from build123d import *

# Parameters (mm, degrees)
SKETCH1_W           = 100
SKETCH1_H           = 8
BOSS_EXTRUDE1_DEPTH = 7
SKETCH3_W           = 100
SKETCH3_H           = 20
BOSS_EXTRUDE2_DEPTH = 2
SKETCH2_W           = 100
SKETCH2_H           = 3.1
CUT_EXTRUDE1_DEPTH  = 5.7
FILLET1_R           = 1
SKETCH4_R           = 2.1
CUT_EXTRUDE2_DEPTH  = 2
FILLET2_R           = 0.75
CHAMFER1_SIZE       = 0.75


with BuildPart() as part:
    # Sketch1 → Boss-Extrude1 (new body)
    with BuildSketch(Plane(origin=(0, 0, 0), x_dir=(1, 0, 0), z_dir=(0, 1, 0))):
        Rectangle(SKETCH1_W, SKETCH1_H)
    extrude(amount=BOSS_EXTRUDE1_DEPTH)

    # Sketch3 → Boss-Extrude2 (add)
    with BuildSketch(Plane(origin=(0, 0, 0), x_dir=(1, 0, 0), z_dir=(0, 1, 0))):
        Rectangle(SKETCH3_W, SKETCH3_H)
    extrude(amount=BOSS_EXTRUDE2_DEPTH)

    # Sketch2 → Cut-Extrude1 (cut)
    with BuildSketch(Plane(origin=(0, 7, 0), x_dir=(1, 0, 0), z_dir=(0, 1, 0))):
        Rectangle(SKETCH2_W, SKETCH2_H)
    extrude(amount=-CUT_EXTRUDE1_DEPTH, mode=Mode.SUBTRACT)

    # Fillet1
    fillet1_edges = [part.edges().sort_by_distance(p)[0] for p in [
        (-50, 7, -2.775),
        (0, 7, 4),
        (50, 7, -2.775),
        (-50, 7, 2.775),
        (0, 7, -1.55),
        (0, 7, 1.55),
        (50, 7, 2.775),
        (0, 7, -4),
    ]]
    fillet(fillet1_edges, radius=FILLET1_R)

    # Sketch4 → Cut-Extrude2 (cut)
    with BuildSketch(Plane(origin=(0, 2, 0), x_dir=(1, 0, 0), z_dir=(0, 1, 0))):
        with Locations(Location((-45.9, 7, 0), (0, 0, 270))):
            Circle(SKETCH4_R)
        with Locations(Location((-45.9, -7, 0), (0, 0, 270))):
            Circle(SKETCH4_R)
        with Locations(Location((45.9, 7, 0), (0, 0, 270))):
            Circle(SKETCH4_R)
        with Locations(Location((45.9, -7, 0), (0, 0, 270))):
            Circle(SKETCH4_R)
    extrude(amount=-CUT_EXTRUDE2_DEPTH, mode=Mode.SUBTRACT)

    # Fillet2
    fillet2_edges = [part.edges().sort_by_distance(p)[0] for p in [
        (-50, 2, -7),
        (50, 2, -7),
        (0, 2, -10),
        (50, 2, 7),
        (-50, 2, 7),
        (0, 2, 10),
    ]]
    fillet(fillet2_edges, radius=FILLET2_R)

    # Chamfer1
    # the kernel refuses this chamfer: 0.75 mm, written as the material it adds along each edge
    with BuildSketch(Plane(origin=(49.25, 2, -4), x_dir=(0, -0.02749587661058648, -0.9996219169112968), z_dir=(-1, 0, 0)), Plane(origin=(-49.25, 2, 4), x_dir=(0, -0.02749587661058648, 0.9996219169112968), z_dir=(1, 0, 0))) as chamfer1_piece_1:
        Polygon((CHAMFER1_SIZE * 0.999621916911, -CHAMFER1_SIZE * 0.0274958766106), (-CHAMFER1_SIZE * 0.0274958766106, -CHAMFER1_SIZE * 0.999621916911), (0, 0), align=None)
    extrude(amount=98.5)
    with BuildSketch(Plane(origin=(49.25, 1.25, -4), x_dir=(-0.8425066666450713, -0.5386859165215022, 0), z_dir=(-0.5386859165215022, 0.8425066666450713, 0))) as chamfer1_piece_2_section:
        Polygon((0.75, -CHAMFER1_SIZE), (0.75 + CHAMFER1_SIZE, 0), (0.75, 0), align=None)
    chamfer1_piece_2 = revolve(axis=Axis((49.25, 1.25, -4), (0, 0, 1)), revolution_arc=237.405771779, mode=Mode.PRIVATE)
    chamfer1_piece_2 = split(chamfer1_piece_2, bisect_by=Plane(origin=(50, 1.825736319, -4.33178547), z_dir=(-1, 0, 0)), keep=Keep.TOP, mode=Mode.PRIVATE)
    chamfer1_piece_2 = split(chamfer1_piece_2, bisect_by=Plane(origin=(49.825736319, 0, -4.33178547), z_dir=(0, 1, 0)), keep=Keep.TOP, mode=Mode.PRIVATE)
    add(chamfer1_piece_2)
    with BuildSketch(Plane(origin=(49.25, 1.25, 4), x_dir=(-0.8425066666450713, -0.5386859165215022, 0), z_dir=(-0.5386859165215022, 0.8425066666450713, 0))) as chamfer1_piece_3_section:
        Polygon((0.75 + CHAMFER1_SIZE, 0), (0.75, CHAMFER1_SIZE), (0.75, 0), align=None)
    chamfer1_piece_3 = revolve(axis=Axis((49.25, 1.25, 4), (0, 0, 1)), revolution_arc=237.405771779, mode=Mode.PRIVATE)
    chamfer1_piece_3 = split(chamfer1_piece_3, bisect_by=Plane(origin=(50, 1.825736319, 4.33178547), z_dir=(-1, 0, 0)), keep=Keep.TOP, mode=Mode.PRIVATE)
    chamfer1_piece_3 = split(chamfer1_piece_3, bisect_by=Plane(origin=(49.825736319, 0, 4.33178547), z_dir=(0, 1, 0)), keep=Keep.TOP, mode=Mode.PRIVATE)
    add(chamfer1_piece_3)
    with BuildSketch(Plane(origin=(-49.25, 1.25, 4), x_dir=(0, 1, 0), z_dir=(1, 0, 0))) as chamfer1_piece_4_section:
        Polygon((0.75, CHAMFER1_SIZE), (0.75 + CHAMFER1_SIZE, 0), (0.75, 0), align=None)
    chamfer1_piece_4 = revolve(axis=Axis((-49.25, 1.25, 4), (0, 0, 1)), revolution_arc=237.405771779, mode=Mode.PRIVATE)
    chamfer1_piece_4 = split(chamfer1_piece_4, bisect_by=Plane(origin=(-50, 1.825736319, 4.33178547), z_dir=(1, 0, 0)), keep=Keep.TOP, mode=Mode.PRIVATE)
    chamfer1_piece_4 = split(chamfer1_piece_4, bisect_by=Plane(origin=(-49.825736319, 0, 4.33178547), z_dir=(0, 1, 0)), keep=Keep.TOP, mode=Mode.PRIVATE)
    add(chamfer1_piece_4)
    with BuildSketch(Plane(origin=(-49.25, 1.25, -4), x_dir=(0, 1, 0), z_dir=(1, 0, 0))) as chamfer1_piece_5_section:
        Polygon((0.75, -CHAMFER1_SIZE), (0.75 + CHAMFER1_SIZE, 0), (0.75, 0), align=None)
    chamfer1_piece_5 = revolve(axis=Axis((-49.25, 1.25, -4), (0, 0, 1)), revolution_arc=237.405771779, mode=Mode.PRIVATE)
    chamfer1_piece_5 = split(chamfer1_piece_5, bisect_by=Plane(origin=(-50, 1.825736319, -4.33178547), z_dir=(1, 0, 0)), keep=Keep.TOP, mode=Mode.PRIVATE)
    chamfer1_piece_5 = split(chamfer1_piece_5, bisect_by=Plane(origin=(-49.825736319, 0, -4.33178547), z_dir=(0, 1, 0)), keep=Keep.TOP, mode=Mode.PRIVATE)
    add(chamfer1_piece_5)


solid = part.part
Source: CAD feature listing. Evaluate the final solid. Frame: model axes, mm. A direction names the side the tool comes from. Give positions to 0.01 mm unless a question says otherwise; leave off trailing zeros. Write each loop counter-clockwise with the first axis right and the second up, starting at its lowest first coordinate (ties: lowest second). Pieces come first, ordered by that corner, then holes. Notation, with made-up numbers: (25, 19) -> (75, 19) arc R31 ccw to (75, 54) -> close; hole circle Ø11 at (24, 51). An arc over 180 degrees is marked (long way). Return JSON: item names as keys, results as strings. Group by question number.
1. Mould query, pull axis X, two halves, no side actions, for faces 1 (the face through (48, 1, 7)), 2 (the face through (-1, 2, -7)), 3 (the face through (48, 1, -7)), 4 (the face through (50, 1, 0)). Classes: +X half, -X half, draft (parallel to the pull), parting line (faces both ways), or undercut.
2. Material intervals for line 1 (X direction, y = 1.05, z = -7); line 2 (Z direction, x = -10.5, y = 5); line 3 (Y direction, x = 6.5, z = 7.5), sorted ascending. Write a range as from..to.
3. Section C-C, the plane z = 7. Output: boundary loops of the cut face in (x, y), then the cut area to 3 significant figures.
4. Access query for faces 5 (the face through (-1, 4, 1.55)), 6 (the face through (-1, 2, 7)), 7 (the face through (1, 0, 0)). Directions: +Z, -Z, +X, -X, +Y, -Y. A direction counts if a zero-diameter tool reaches every point of the face in a straight line with its end or side. Return the directions, or none.
5. Section D-D, the plane x = 11.5. Output: boundary loops of the cut face in (y, z), then the cut area to 3 significant figures.
6. Section B-B, the plane y = 5. Output: boundary loops of the cut face in (x, z), then the cut area to 3 significant figures.
7. Pin query (flat end, axial travel): pin 1 Ø3.5 at (x, z) = (45.9, 7) entering from -Y; pin 2 Ø1.4 at (x, z) = (8, 7.5) entering from +Y; pin 3 Ø0.9 at (x, z) = (9, 0.5) entering from +Y; pin 4 Ø1.7 at (x, y) = (-22, 4.5) entering from +Z. Return the tip coordinate at first contact, or that it passes through.
8. Section A-A, the plane x = 45.9. Output: boundary loops of the cut face in (y, z), then the cut area to 3 significant figures.
Determined:
{
 "1": {"face 1": "undercut", "face 2": "draft", "face 3": "undercut", "face 4": "+X half"},
 "2": {"line 1": "x = -50..-48, -43.8..43.8, 48..50", "line 2": "z = -4..-1.55, 1.55..4", "line 3": "y = 0..2"},
 "3": {"outline": "(-50, 0) -> (-48, 0) -> (-48, 2) -> (-49.25, 2) arc R0.75 ccw to (-50, 1.25) -> close; (-43.8, 0) -> (43.8, 0) -> (43.8, 2) -> (-43.8, 2) -> close; (48, 0) -> (50, 0) -> (50, 1.25) arc R0.75 ccw to (49.25, 2) -> (48, 2) -> close", "area": "183 mm2"},
 "4": {"face 5": "+X, -X, +Y", "face 6": "+Z, +X, -X, +Y", "face 7": "+Z, -Z, +X, -X, -Y"},
 "5": {"outline": "(0, -10) -> (1.25, -10) arc R0.75 ccw to (2, -9.25) -> (2, -4.75) -> (2.75, -4) -> (6, -4) arc R1 ccw to (7, -3) -> (7, -2.55) arc R1 ccw to (6, -1.55) -> (1.3, -1.55) -> (1.3, 1.55) -> (6, 1.55) arc R1 ccw to (7, 2.55) -> (7, 3) arc R1 ccw to (6, 4) -> (2.75, 4) -> (2, 4.75) -> (2, 9.25) arc R0.75 ccw to (1.25, 10) -> (0, 10) -> close", "area": "61.8 mm2"},
 "6": {"outline": "(-50, -4) -> (50, -4) -> (50, -1.55) -> (-50, -1.55) -> close; (-50, 1.55) -> (50, 1.55) -> (50, 4) -> (-50, 4) -> close", "area": "490 mm2"},
 "7": {"pin 1": "passes through", "pin 2": "stops at y = 2", "pin 3": "stops at y = 1.3", "pin 4": "stops at z = 4"},
 "8": {"outline": "(0, -10) -> (1.25, -10) arc R0.75 ccw to (2, -9.25) -> (2, -9.1) -> (0, -9.1) -> close; (0, -4.9) -> (2, -4.9) -> (2, -4.75) -> (2.75, -4) -> (6, -4) arc R1 ccw to (7, -3) -> (7, -2.55) arc R1 ccw to (6, -1.55) -> (1.3, -1.55) -> (1.3, 1.55) -> (6, 1.55) arc R1 ccw to (7, 2.55) -> (7, 3) arc R1 ccw to (6, 4) -> (2.75, 4) -> (2, 4.75) -> (2, 4.9) -> (0, 4.9) -> close; (0, 9.1) -> (2, 9.1) -> (2, 9.25) arc R0.75 ccw to (1.25, 10) -> (0, 10) -> close", "area": "45.0 mm2"}
}
